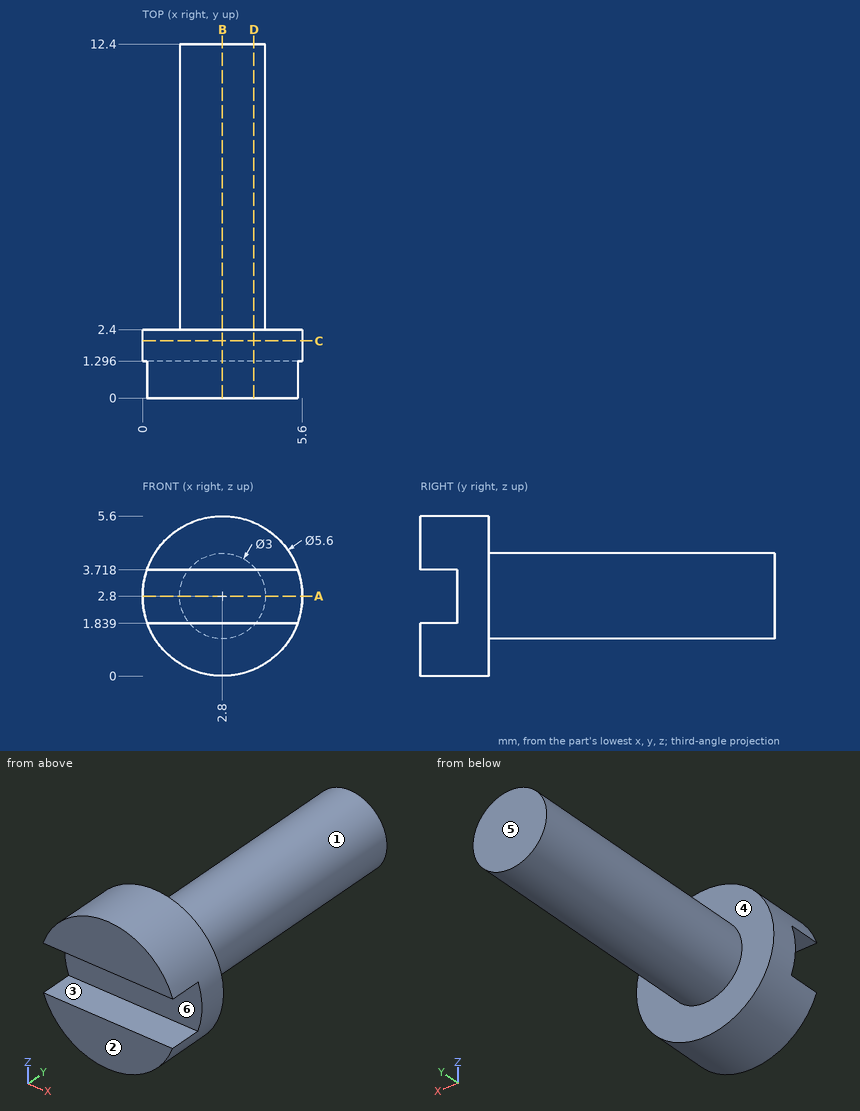
Input: dimensioned drawing with shaded views. Units: mm. Origin: part minimum x, y, z. A direction names the side the tool comes from. Coordinates: 2 decimals unless noted, no trailing zeros. Order: outer loops, then holes, each group sorted by start corner. A loop starts at its lowest first (then second) coordinate and runs counter-clockwise, first axis right, second up.
Item 1: Draft query along Z for the marked faces 1, 2 and 3. Return one class per face: released by +Z, released by -Z, zero draft, split by the parting line, or undercut.
Answer:
face 1: split by the parting line
face 2: zero draft
face 3: undercut
Item 2: Section query C-C (y = 2). Output: boundary loops of the cut face in (x, z).
Answer:
outline: circle Ø5.6 at (2.8, 2.8)
Item 3: Material intervals for line 1 along Z through (x, y) = (0.3, 0.5) (1 decimal); line 2 along Y through (x, z) = (4, 3.1); line 3 along Y through (x, z) = (4.1, 1.5), sorted ascending.
Answer:
line 1: z = 1.5 to 1.8, 3.7 to 4.1
line 2: y = 1.3 to 12.4
line 3: y = 0 to 2.4
Item 4: Section query D-D (x = 3.9). Output: boundary loops of the cut face in (y, z) (1 decimal).
Answer:
outline: (0, 0.2) - (2.4, 0.2) - (2.4, 1.8) - (12.4, 1.8) - (12.4, 3.8) - (2.4, 3.8) - (2.4, 5.4) - (0, 5.4) - (0, 3.7) - (1.3, 3.7) - (1.3, 1.8) - (0, 1.8) - close
Item 5: Section query A-A (z = 2.8). Output: boundary loops of the cut face in (x, y).
Answer:
outline: (0, 1.3) - (5.6, 1.3) - (5.6, 2.4) - (4.3, 2.4) - (4.3, 12.4) - (1.3, 12.4) - (1.3, 2.4) - (0, 2.4) - close
Item 6: Access query for the marked faces 4, 5 and 6. Directions: +Z, -Z, +X, -X, +Y, -Y. A direction counts if a zero-diameter tool reaches every point of the face in a straight line with its end or side. Return the directions, or none.
Answer:
face 4: +Y
face 5: +Z, -Z, +X, -X, +Y
face 6: +X, -X, -Y
Item 7: Section query B-B (x = 2.8). Output: boundary loops of the cut face in (y, z), then the cut area to 3 significant figures.
Answer:
outline: (0, 0) - (2.4, 0) - (2.4, 1.3) - (12.4, 1.3) - (12.4, 4.3) - (2.4, 4.3) - (2.4, 5.6) - (0, 5.6) - (0, 3.72) - (1.3, 3.72) - (1.3, 1.84) - (0, 1.84) - close
area: 41.0 mm2
Item 8: Contact query for flat-ended pins moving along their axis: P1, Ø0.6, axis at x = 4, z = 3, coming from the -Y side; P2, Ø1.5, axis at x = 1, y = 6, coming from the +Z side; P3, Ø1, axis at y = 8, z = 4, coming from the -X side. Output: stop coordinate, or through.
Answer:
P1: stops at y = 1.3
P2: stops at z = 3.87
P3: stops at x = 1.47
